Autodesk Inventor part; units mm, degrees
ref_plane "YZ Plane" through (0, 0, 0) normal (1, 0, 0) x (0, 1, 0)
ref_plane "XZ Plane" through (0, 0, 0) normal (0, 1, 0) x (-1, 0, 0)
ref_plane "XY Plane" through (0, 0, 0) normal (0, 0, 1) x (1, 0, 0)
sketch "Sketch1" plane through (0, 0, 0) normal (0, 0, 1) x (1, 0, 0)
  circle A0 centre (0, 0) radius 12.5
  dimension "d0" = 25
extrude "Extrusion1" add sketch "Sketch1" along normal blind 52
sketch "Sketch2" plane through (0, 0, 0) normal (0, 0, -1) x (-1, 0, 0)
  circle A0 centre (0, 0) radius 3.5
  dimension "d3" = 7
extrude "Extrusion2" add sketch "Sketch2" along normal blind 2.5
sketch "Sketch3" plane through (0, 0, -2.5) normal (0, 0, -1) x (-1, 0, 0)
  circle A0 centre (0, 0) radius 2.5
  dimension "d6" = 5
extrude "Extrusion3" add sketch "Sketch3" along normal blind 9
sketch "Sketch4" plane through (0, 0, -11.5) normal (0, 0, -1) x (-1, 0, 0)
  line L0 (2, -1.5) -> (-2, -1.5)
  circle A0 centre (0, 0) radius 2.5
  dimension "d9" = 1.5
extrude "Extrusion4" cut sketch "Sketch4" against normal blind 8 contours A0 L0 picked at (-0.534, -1.6398)
sketch "Sketch5" plane through (0, 0, 0) normal (0, 0, -1) x (-1, 0, 0)
  circle A0 centre (0, -8.5) radius 1.5
  circle A1 centre (0, 8.5) radius 1.5
  point P0 (0, 0)
  dimension "d12" = 3
  dimension "d13" = 8.5
  dimension "d14" = 3
  dimension "d15" = 17
extrude "Extrusion5" cut sketch "Sketch5" against normal blind 3
properties part number "Motor" material "Stainless Steel"
Check sheet for the modelled part. Datum: model origin and axes. Units: mm. A direction names the side the tool comes from. Round coordinates to 2 decimals unless told otherwise and drop trailing zeros. Order: outer loops, then holes, each group sorted by start corner. A loop starts at its lowest first (then second) coordinate and runs counter-clockwise, first axis right, second up. Notation, with made-up numbers: M -7.75,87.25 L 0.25,87.25 A13 cw 0.25,93.25 Z; hole C 4.25,-27.5 d6. An arc over 180 degrees is marked long. Answer in a Markdown table with one row per item.
(1) Section check D-D on y = 8.5. Record the boundary of the cut face in (x, z), plus the area to 3 significant figures.
Findings:
| item | result |
|---|---|
| outline | M -9.17,0 L -1.5,0 L -1.5,3 L 1.5,3 L 1.5,0 L 9.17,0 L 9.17,52 L -9.17,52 Z |
| area | 944 mm^2 |
(2) Set-up check for faces 1 (the cylindrical face through (-3.233, 1.341, -1.232)), 2 (the cylindrical face through (11.923, -3.755, 25.636)): record each of +Z, -Z, +X, -X, +Y, -Y from which the full face is reachable in a straight line by a thin tool's end or side.
Findings:
| item | result |
|---|---|
| face 1 | -Z |
| face 2 | +Z, -Z |
(3) Draft check along Y on faces 3 (the flat face through (-2, -2, -2.5)), 4 (the flat face through (0, 9, 3)), 5 (the flat face through (0, -1.5, -8)). Enter one of: +Y half, -Y half, draft (parallel to the pull), parting line (faces both ways), or undercut.
Findings:
| item | result |
|---|---|
| face 3 | draft |
| face 4 | undercut |
| face 5 | -Y half |
(4) Section check C-C on z = 35. Record the boundary of the cut face in (x, y), plus the area to 3 significant figures.
Findings:
| item | result |
|---|---|
| outline | C 0,0 d25 |
| area | 491 mm^2 |
(5) Section check B-B on x = 0. Record the boundary of the cut face in (y, z), plus the area to 3 significant figures.
Findings:
| item | result |
|---|---|
| outline | M -12.5,0 L -10,0 L -10,3 L -7,3 L -7,0 L -3.5,0 L -3.5,-2.5 L -2.5,-2.5 L -2.5,-3.5 L -1.5,-3.5 L -1.5,-11.5 L 2.5,-11.5 L 2.5,-2.5 L 3.5,-2.5 L 3.5,0 L 7,0 L 7,3 L 10,3 L 10,0 L 12.5,0 L 12.5,52 L -12.5,52 Z |
| area | 1,340 mm^2 |
(6) Material ranges on line 1 along Y through (x, z) = (0, 2.1); line 2 along Y through (x, z) = (-7.5, 19.5); line 3 along Z through (x, y) = (4, -7.25), recorded low to high. Write a range as from..to.
Findings:
| item | result |
|---|---|
| line 1 | y = -12.5..-10, -7..7, 10..12.5 |
| line 2 | y = -10..10 |
| line 3 | z = 0..52 |
(7) Section check A-A on y = 0. Record the boundary of the cut face in (x, z).
Findings:
| item | result |
|---|---|
| outline | M -12.5,0 L -3.5,0 L -3.5,-2.5 L -2.5,-2.5 L -2.5,-11.5 L 2.5,-11.5 L 2.5,-2.5 L 3.5,-2.5 L 3.5,0 L 12.5,0 L 12.5,52 L -12.5,52 Z |
(8) Gauge pin test, flat ends, axial feed: pin 1 (6 mm diameter, centred on x = -8.5, z = 40.5, fed in from +Y) (3 decimals); pin 2 (1 mm diameter, centred on x = -0.5, y = -6.5, fed in from -Z); pin 3 (0.8 mm diameter, centred on x = 0.5, y = -2, fed in from -Z). Record the tip position at first contact, or that the pin passes through.
Findings:
| item | result |
|---|---|
| pin 1 | stops at y = 11.225 |
| pin 2 | stops at z = 0 |
| pin 3 | stops at z = -3.5 |
